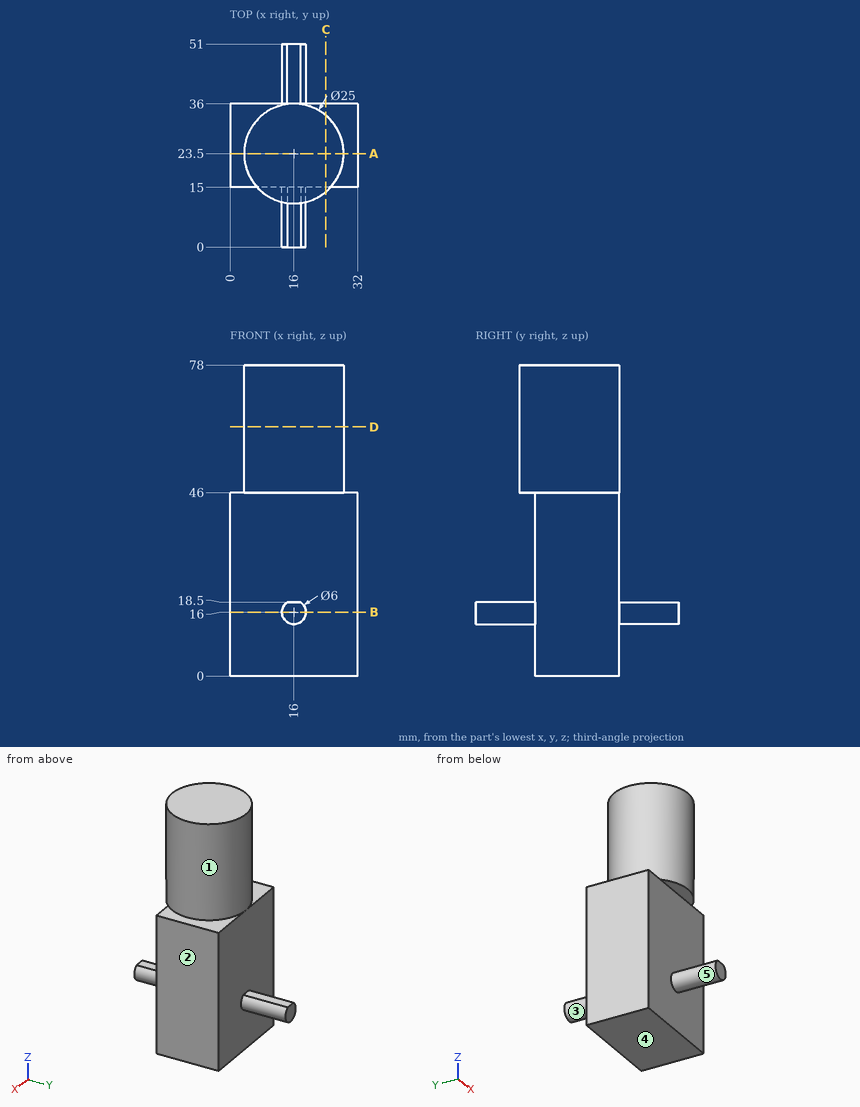
Design review of the part shown in the three views and the two pictorial views. Dimensions are in mm from the part's minimum x, y and z. A direction names the side the tool comes from. Round coordinates to 2 decimals unless told otherwise and drop trailing zeros. Write each loop counter-clockwise with the first axis right and the second up, starting at its lowest first coordinate (ties: lowest second). Pieces come first, ordered by that corner, then holes. Notation, with made-up numbers: M -2.5,23.5 L 42.5,23.5 A31 cw 42.5,48.5 Z; hole C 0.5,65.25 d4. An arc over 180 degrees is marked long. One line per item, written item: value. Start each with the question number.
1. Take a section at C-C on x = 24. State the section outline as (y, z) points, then the cut area to 3 significant figures.
2. To check wall thickness, follow probe 1 along Z at (x, y) = (16, 14); probe 2 along Y at (x, z) = (23, 31); probe 3 along Z at (x, y) = (20, 14). State the ranges of each line that lie inside material, in increasing order. Write a range as from..to.
3. For the marked faces 1, 2, 3, 4 and 5, list the 3-axis set-ups (+Z, -Z, +X, -X, +Y, -Y) from which the entire face can be reached by the end or side of a thin tool; tool diameter is ignored.
4. Take a section at B-B on z = 16. State the section outline as (x, y) points.
5. Clearance check with flat-ended pins moving along their axes: P1, Ø2.5, axis at x = 16.5, y = 9.5, coming from the +Z side; P2, Ø5, axis at x = 27, z = 33, coming from the +Y side; P3, Ø1, axis at y = 35.5, z = 59, coming from the -X side. State where each tip first meets the part, or that it passes through.
6. Take a section at A-A on y = 23.5. State the section outline as (x, z) points.
7. Take a section at D-D on z = 62.5. State the section outline as (x, y) points.
Computed:
1. outline: M 13.9,46 L 15,46 L 15,0 L 36,0 L 36,46 L 33.1,46 L 33.1,78 L 13.9,78 Z
1. area: 1,580 mm²
2. probe 1: z = 13..18.5, 46..78
2. probe 2: y = 15..36
2. probe 3: z = 46..78
3. face 1: +Z
3. face 2: +Z, -Z, +X, +Y, -Y
3. face 3: +Y
3. face 4: -Z, +X, -X, +Y, -Y
3. face 5: -Y
4. outline: M 0,15 L 13,15 L 13,0 L 19,0 L 19,15 L 32,15 L 32,36 L 19,36 L 19,51 L 13,51 L 13,36 L 0,36 Z
5. P1: stops at z = 18.5
5. P2: stops at y = 36
5. P3: stops at x = 11.1
6. outline: M 0,0 L 32,0 L 32,46 L 28.5,46 L 28.5,78 L 3.5,78 L 3.5,46 L 0,46 Z
7. outline: C 16,23.5 d25
